from build123d import *

# Parameters (mm, degrees)
F1_DEPTH = 7.366
F2_R     = 14.7883109898
F4_DEPTH = 8.382
F3_R     = 13.603757009
F5_DEPTH = 8.128
F7_DEPTH = 10.922


with BuildPart() as f1:
    # F0 (on Front) → F1 (new body)
    with BuildSketch(Plane.XZ):
        Polygon((-76.4300598123, 62.2463936663), (-137.2705996037, 58.215200901), (-137.2705996037, -72.0348134637), (137.2705996037, -72.0348134637), (140.6780183315, 76.6316130757), (45.3754555261, 70.3170241025), (45.3754555261, 8.0706304363), (-76.4300598123, 0), align=None)
    extrude(amount=F1_DEPTH)

    # F2 (on face) → F4 (join)
    with BuildSketch(Plane(origin=(138.8486896806, 0, -3.1823972404), x_dir=(0, 1, 0), z_dir=(0.9997374427, 0, -0.0229138761))):
        Polygon((122.0736131072, 79.834971573), (0, 79.834971573), (0, -68.8704986774), (122.0736131072, -67.0348182321), align=None)
        with Locations((56.3235022128, 0)):
            Circle(F2_R, mode=Mode.SUBTRACT)
    extrude(amount=-F4_DEPTH)

    # F3 (on face) → F5 (join)
    with BuildSketch(Plane(origin=(-137.2705996037, 0, 0), x_dir=(0, -1, 0), z_dir=(-1, 0, 0))):
        Polygon((0, -72.0348134637), (0, 58.215200901), (-119.2674264312, 58.215200901), (-119.2674264312, -78.3181233552), align=None)
        with Locations((-67.8130164742, -22.7041952312)):
            Circle(F3_R, mode=Mode.SUBTRACT)
    extrude(amount=-F5_DEPTH)

    # F6 (on face) → F7 (join)
    with BuildSketch(Plane(origin=(0, 122.0736131072, 0), x_dir=(-1, 0, 0), z_dir=(0, 1, 0))):
        Polygon((-132.2982190871, 76.8236771856), (-128.9328629136, -70.0075508798), (136.390298605, -77.0845785737), (134.340301156, 58.1577047706), (70.8223407273, 62.6042659656), (70.8223407273, -9.0142149687), (-57.9433558552, 0), (-57.9433558552, 71.6184809343), align=None)
    extrude(amount=-F7_DEPTH)


solid = f1.part
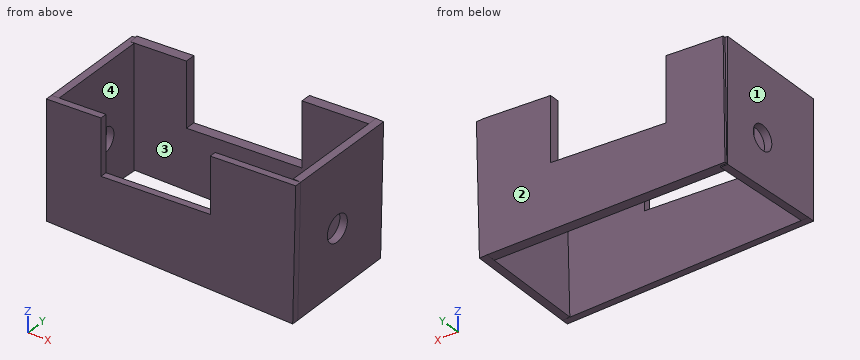
Build history of the part. All positions in model axes, mm. Face numbers are marked on the shaded views. Coordinates: 2 decimals unless noted, no trailing zeros. Write each loop counter-clockwise with the first axis right and the second up, starting at its lowest first coordinate (ties: lowest second). Pieces come first, ordered by that corner, then holes. Notation, with made-up numbers: (66, 63) -> (93, 63) arc R9 cw to (93, 78) -> close; hole circle Ø3 at (81, 11). An arc over 180 degrees is marked (long way). Use CSV: the item, a comma, the result in double quotes. Start each with the question number.
Q1. Cut at B-B, the plane z = 24. List the corners of the cut face in (x, y).
Q2. Cut at C-C, the plane y = 105. List the corners of the cut face in (x, z).
Q3. Flat gauge pins, fed straight in: pin 1 Ø22 at (y, z) = (67.81, -22.7) entering from -X (3 decimals); pin 2 Ø2 at (y, z) = (102.5, -46.5) entering from +X; pin 3 Ø3.5 at (y, z) = (-4, 27.5) entering from +X; pin 4 Ø12 at (y, z) = (119.5, 32) entering from -X. Where does each tip first touch, or does it go through?
Q4. Drill centre lines: probe 1 along Y at (x, z) = (-4.5, -67); probe 2 along Y at (x, z) = (-38, -5.5); probe 3 along X at (y, z) = (94.5, -11). Where is each one in solid material? Low to high.
Q5. Cut at A-A, the plane x = 116.5. List the corners of the cut face in (y, z), then the cut area to 3 significant figures.
Q6. Pull direction X, two halves, no side cores. Call the marked faces 1, 2, 3 and 4: released by +X, released by -X, zero draft, split by the parting line, or undercut.
Q7. Cut at D-D, the plane y = 61. List the corners of the cut face in (x, z), then the cut area to 3 significant figures.
Checked values:
1,outline,"(-137.27, -7.37) -> (-76.43, -7.37) -> (-76.43, 0) -> (-129.14, 0) -> (-129.14, 111.15) -> (-70.82, 111.15) -> (-70.82, 122.07) -> (-134.86, 122.07) -> (-134.86, 119.27) -> (-137.27, 119.27) -> close; (45.38, -7.37) -> (139.47, -7.37) -> (139.47, 122.07) -> (57.94, 122.07) -> (57.94, 111.15) -> (131.09, 111.15) -> (131.09, 0) -> (45.38, 0) -> close"
2,outline,"(-137.27, -77.57) -> (-129.14, -77.57) -> (-129.14, 58.22) -> (-137.27, 58.22) -> close; (128.93, -70.26) -> (137.31, -70.46) -> (140.68, 76.63) -> (132.3, 76.82) -> close"
3,pin 1,"stops at x = 129.765"
3,pin 2,"stops at x = 137.88"
3,pin 3,"stops at x = 139.59"
3,pin 4,"stops at x = -137.27"
4,probe 1,"y = -7.37 to 0, 111.15 to 122.07"
4,probe 2,"y = -7.37 to 0"
4,probe 3,"x = -137.27 to -129.14, 130.29 to 138.67"
5,outline,"(-7.37, -72.03) -> (0, -72.03) -> (0, 75.03) -> (-7.37, 75.03) -> close; (111.15, -70.34) -> (122.07, -70.34) -> (122.07, 75.72) -> (111.15, 75.72) -> close"
5,area,"2,680 mm²"
6,face 1,"released by -X"
6,face 2,"zero draft"
6,face 3,"undercut"
6,face 4,"undercut"
7,outline,"(-137.27, -75.25) -> (-129.14, -75.25) -> (-129.14, -34.48) -> (-137.27, -34.48) -> close; (-137.27, -10.93) -> (-129.14, -10.93) -> (-129.14, 58.22) -> (-137.27, 58.22) -> close; (128.91, -70.93) -> (137.29, -71.12) -> (138.53, -17.21) -> (130.15, -17.02) -> close; (130.79, 11.04) -> (139.17, 10.84) -> (140.68, 76.63) -> (132.3, 76.82) -> close"
7,area,"1,900 mm²"
